For this review, take the finished solid that the model builds, in its own axes (mm). Give positions to 0.01 mm unless a question says otherwise; leave off trailing zeros. Loops run counter-clockwise (first coordinate to the right, second up) from the corner with the lowest first, then second, coordinate; pieces in that order, holes last. Notation, with made-up numbers: (18, 44) - (26, 44) arc R5 ccw to (26, 50) - close; hole circle Ø5 at (73, -29.5). An arc over 180 degrees is marked (long way). Put each result on its own line as item: value. Start each with the question number.
from build123d import *

# Parameters (mm, degrees)
F1_DEPTH = 6.35
F3_D     = 6.35
F4_R     = 5.08
F5_R     = 2.54
F7_D     = 6.35


with BuildPart() as f1:
    # F0 (on Top) → F1 (new body, symmetric)
    with BuildSketch(Plane.XY):
        Polygon((-12.7, 38.1), (-38.1, 12.7), (-38.1, -12.7), (-12.7, -38.1), (12.7, -38.1), (38.1, -12.7), (38.1, 12.7), (12.7, 38.1), align=None)
    extrude(amount=F1_DEPTH, both=True)

    # F3 (through all)
    with Locations(Plane(origin=(-38.1, 0, 0), x_dir=(0, -1, 0), z_dir=(-1, 0, 0))):
        with Locations((0, 0)):
            Hole(F3_D / 2)

    # F4
    f4_edges = [f1.edges().sort_by_distance(p)[0] for p in [
        (-12.7, 38.1, 0),
        (-38.1, 12.7, 0),
        (12.7, 38.1, 0),
        (38.1, 12.7, 0),
        (-38.1, -12.7, 0),
        (-12.7, -38.1, 0),
        (12.7, -38.1, 0),
        (38.1, -12.7, 0),
    ]]
    fillet(f4_edges, radius=F4_R)

    # F5
    f5_edges = [f1.edges().sort_by_distance(p)[0] for p in [
        (-25.4, 25.4, 6.35),
        (-12.539827, 37.713308, 6.35),
        (-37.713308, 12.539827, 6.35),
        (0, 38.1, 6.35),
        (-38.1, 0, 6.35),
        (12.539827, 37.713308, 6.35),
        (-37.713308, -12.539827, 6.35),
        (25.4, 25.4, 6.35),
        (-25.4, -25.4, 6.35),
        (37.713308, 12.539827, 6.35),
        (-12.539827, -37.713308, 6.35),
        (38.1, 0, 6.35),
        (0, -38.1, 6.35),
        (37.713308, -12.539827, 6.35),
        (12.539827, -37.713308, 6.35),
        (25.4, -25.4, 6.35),
        (-25.4, 25.4, -6.35),
        (-12.539827, 37.713308, -6.35),
        (-37.713308, 12.539827, -6.35),
        (0, 38.1, -6.35),
        (-38.1, 0, -6.35),
        (12.539827, 37.713308, -6.35),
        (-37.713308, -12.539827, -6.35),
        (25.4, 25.4, -6.35),
        (-25.4, -25.4, -6.35),
        (37.713308, 12.539827, -6.35),
        (-12.539827, -37.713308, -6.35),
        (38.1, 0, -6.35),
        (0, -38.1, -6.35),
        (37.713308, -12.539827, -6.35),
        (12.539827, -37.713308, -6.35),
        (25.4, -25.4, -6.35),
    ]]
    fillet(f5_edges, radius=F5_R)

    # F7 (through all)
    with Locations(Plane(origin=(0, 38.1, 0), x_dir=(-1, 0, 0), z_dir=(0, 1, 0))):
        with Locations((0, 0)):
            Hole(F7_D / 2)


solid = f1.part
1) Mouldability with a two-part tool opening along X and no side actions: class faces 1 (the cylindrical face through (24.73, 25.04, -5.59)), 2 (the cylindrical face through (-0.41, -19.32, 3.15)), 3 (the flat face through (-38.1, 0.15, -3.33)) as released by +X, released by -X, zero draft, split by the parting line, or undercut.
2) Insertion check: P1, Ø1.5, axis at x = 29.5, z = 3.5, coming from the -Y side; P2, Ø4, axis at x = 0, z = 0, coming from the -Y side; P3, Ø2, axis at x = 17.5, z = -3, coming from the -Y side; P4, Ø6, axis at y = 17, z = 3, coming from the -X side. Each pin has a flat end and moves straight along its axis. Give the tip position at first contact, or say it passes through.
3) Wall thickness on probe 1 along X at (y, z) = (-10, 0) (3 decimals); probe 2 along Z at (x, y) = (25.5, 0) (3 decimals): over which ranges is each line inside the solid? List them lowest first.
4) Take a section at A-A on z = 0. State the section outline as (x, y) points (3 decimals).
5) Take a section at B-B on x = -4.5. State the section outline as (y, z) points (3 decimals), and give its area (3 significant figures).
Answers follow:
1. face 1: released by +X
1. face 2: undercut
1. face 3: released by -X
2. P1: y = -22.05
2. P2: through
2. P3: y = -34.3
2. P4: x = -36.79
3. probe 1: -38.1 to -3.175, 3.175 to 38.1
3. probe 2: -6.35 to -3.175, 3.175 to 6.35
4. outline: (-38.1, -10.596) arc R5.08 ccw to (-36.612, -14.188) - (-14.188, -36.612) arc R5.08 ccw to (-10.596, -38.1) - (-3.175, -38.1) - (-3.175, -3.175) - (-38.1, -3.175) - close; (-38.1, 3.175) - (-3.175, 3.175) - (-3.175, 38.1) - (-10.596, 38.1) arc R5.08 ccw to (-14.188, 36.612) - (-36.612, 14.188) arc R5.08 ccw to (-38.1, 10.596) - close; (3.175, -38.1) - (10.596, -38.1) arc R5.08 ccw to (14.188, -36.612) - (36.612, -14.188) arc R5.08 ccw to (38.1, -10.596) - (38.1, -3.175) - (3.175, -3.175) - close; (3.175, 3.175) - (38.1, 3.175) - (38.1, 10.596) arc R5.08 ccw to (36.612, 14.188) - (14.188, 36.612) arc R5.08 ccw to (10.596, 38.1) - (3.175, 38.1) - close
5. outline: (-38.1, -3.81) arc R2.54 ccw to (-35.56, -6.35) - (35.56, -6.35) arc R2.54 ccw to (38.1, -3.81) - (38.1, 3.81) arc R2.54 ccw to (35.56, 6.35) - (-35.56, 6.35) arc R2.54 ccw to (-38.1, 3.81) - close; hole circle Ø6.35 at (0, 0)
5. area: 931 mm2
